Geometry: final body of the model. Coordinates: model frame, mm. A direction names the side the tool comes from. Round coordinates to 2 decimals unless told otherwise and drop trailing zeros. Loops run counter-clockwise (first coordinate to the right, second up) from the corner with the lowest first, then second, coordinate; pieces in that order, holes last. Notation, with made-up numbers: (36.25, 46) - (40.25, 46) arc R15 cw to (40.25, 52) - close; hole circle Ø2 at (7.5, 85.25). An arc over 180 degrees is marked (long way). Use CSV: the item, a comma, the result in double quotes.
from build123d import *

# Parameters (mm, degrees)
SKETCH_R     = 10
PAD_DEPTH    = 15
SKETCH001_R  = 15
PAD001_DEPTH = 15
FILLET_R     = 12


with BuildPart() as part:
    # Sketch → Pad (new body)
    with BuildSketch(Plane.XZ):
        with BuildLine():
            ThreePointArc((-76.583116, 18.708294), (-83.37421, -8.868276), (-60, -25))
            Line((-60, -25), (60, -25))
            ThreePointArc((60, -25), (83.374198, -8.868308), (76.583166, 18.70825))
            Line((30, 60), (76.583166, 18.70825))
            Line((-30, 60), (30, 60))
            Line((-76.583116, 18.708294), (-30, 60))
        make_face()
        with Locations((-60, 0)):
            Circle(SKETCH_R, mode=Mode.SUBTRACT)
        with Locations((60, 0)):
            Circle(SKETCH_R, mode=Mode.SUBTRACT)
    extrude(amount=PAD_DEPTH)

    # Sketch001 → Pad001 (new body)
    with BuildSketch(Plane(origin=(0, 0, 60), x_dir=(-1, 0, 0), z_dir=(0, 0, 1))):
        with BuildLine():
            ThreePointArc((30, 44.999961), (2e-05, 75), (-30, 45.000001))
            Line((-30, 0), (-30, 45.000001))
            Line((-30, 0), (30, 0))
            Line((30, 0), (30, 44.999961))
        make_face()
        with Locations((0, 45)):
            Circle(SKETCH001_R, mode=Mode.SUBTRACT)
    extrude(amount=-PAD001_DEPTH)

    # Fillet
    fillet_edges = [part.edges().sort_by_distance(p)[0] for p in [
        (0, -15, 45),
    ]]
    fillet(fillet_edges, radius=FILLET_R)


solid = part.part
Item 1: Section C-C on y = -58. Return the cut outline in (x, z), plus the area to 3 significant figures.
Final values:
outline,"(-27.04, 45) - (-7.48, 45) - (-7.48, 60) - (-27.04, 60) - close; (7.48, 45) - (27.04, 45) - (27.04, 60) - (7.48, 60) - close"
area,"587 mm²"
Item 2: Section D-D on y = -37.5. Return the cut outline in (x, z), plus the area to 3 significant figures.
Final values:
outline,"(-30, 45) - (-12.99, 45) - (-12.99, 60) - (-30, 60) - close; (12.99, 45) - (30, 45) - (30, 60) - (12.99, 60) - close"
area,"510 mm²"
Item 3: Reachability of faces 4 (the flat face through (0, -62, 45)), 5 (the flat face through (-30, -30, 53)), 6 (the flat face through (30, -30, 53)) from +Z, -Z, +X, -X, +Y, -Y: full face, straight path, thin tool, end or side. Return the list, or none.
Final values:
face 4,"-Z, +X, -X, -Y"
face 5,"+Z, -Z, -X, -Y"
face 6,"+Z, -Z, +X, -Y"
Item 4: Pin query (flat end, axial travel): P1, Ø1, axis at x = -18, z = 46.5, coming from the -Y side; P2, Ø8, axis at y = -27, z = 50.5, coming from the -X side; P3, Ø13.5, axis at y = -27, z = 45, coming from the +X side. Return the tip coordinate at first contact, or that it passes through.
Final values:
P1,"stops at y = -69.37"
P2,"stops at x = -30"
P3,"stops at x = 30"
Item 5: Section B-B on x = 7.5. Return the cut outline in (y, z), plus the area to 3 significant figures.
Final values:
outline,"(-74.05, 45) - (-57.99, 45) - (-57.99, 60) - (-74.05, 60) - close; (-32.01, 45) - (-27, 45) arc R12 cw to (-15, 33) - (-15, -25) - (0, -25) - (0, 60) - (-32.01, 60) - close"
area,"1,800 mm²"
Item 6: Section A-A on z = 0. Return the cut outline in (x, y).
Final values:
outline,"(-85, -15) - (-70, -15) - (-70, 0) - (-85, 0) - close; (-50, -15) - (50, -15) - (50, 0) - (-50, 0) - close; (70, -15) - (85, -15) - (85, 0) - (70, 0) - close"
Item 7: Mould query, pull axis Z, two halves, no side actions, for faces 1 (the flat face through (0.4, -29.7, 60)), 2 (the cylindrical face through (-70, -7, 0)), 3 (the flat face through (-1, -15, 9)). Classes: released by +Z, released by -Z, zero draft, split by the parting line, or undercut.
Final values:
face 1,"released by +Z"
face 2,"undercut"
face 3,"zero draft"
Item 8: Material intervals for line 1 (Y direction, x = 0, z = 52); line 2 (X direction, y = -45, z = 48.75); line 3 (Z direction, x = -12, y = -66), sorted ascending.
Final values:
line 1,"y = -75 to -60, -30 to 0"
line 2,"x = -30 to -15, 15 to 30"
line 3,"z = 45 to 60"
